from build123d import *

# Parameters (mm, degrees)
F0_W     = 2
F0_H     = 2
F0_W_2   = 1
F0_W_3   = 21
F1_DEPTH = 25
F2_DEPTH = 1
F3_START = 24
F3_DEPTH = 1
F4_W     = 23
F4_H     = 4.75
F5_DEPTH = 25


with BuildPart() as f1:
    # F0 (on Front) → F1 (new body)
    with BuildSketch(Plane.XZ):
        with BuildLine():
            Line((-12.4285714286, 13.5171716937), (-14.4285714286, 13.5171716937))
            Line((-14.4285714286, 13.5171716937), (-14.4285714286, 2.0171716937))
            ThreePointArc((-14.4285714286, 2.0171716937), (-1.9285714286, -10.4828283063), (10.5714285714, 2.0171716937))
            Line((10.5714285714, 2.0171716937), (10.5714285714, 13.5171716937))
            Line((10.5714285714, 13.5171716937), (8.5714285714, 13.5171716937))
            Line((8.5714285714, 13.5171716937), (8.5714285714, 2.0171716937))
            ThreePointArc((8.5714285714, 2.0171716937), (-1.9285714286, -8.4828283063), (-12.4285714286, 2.0171716937))
            Line((-12.4285714286, 2.0171716937), (-12.4285714286, 13.5171716937))
        make_face()
        with Locations((9.5714285714, 14.5171716937)):
            Rectangle(F0_W, F0_H)
        with Locations((-13.4285714286, 14.5171716937)):
            Rectangle(F0_W, F0_H)
        with Locations((-14.9285714286, 14.5171716937)):
            Rectangle(F0_W_2, F0_H)
        with Locations((-1.9285714286, 14.5171716937)):
            Rectangle(F0_W_3, F0_H)
        with Locations((11.0714285714, 14.5171716937)):
            Rectangle(F0_W_2, F0_H)
    extrude(amount=F1_DEPTH)

    # F0 (on Front) → F2 (join)
    with BuildSketch(Plane.XZ):
        with BuildLine():
            Line((-14.4285714286, 13.5171716937), (-15.4285714286, 13.5171716937))
            Line((-15.4285714286, 13.5171716937), (-15.4285714286, 2.0171716937))
            ThreePointArc((-15.4285714286, 2.0171716937), (-11.4745129746, -7.5287698523), (-1.9285714286, -11.4828283063))
            ThreePointArc((-1.9285714286, -11.4828283063), (7.6173701174, -7.5287698523), (11.5714285714, 2.0171716937))
            Line((11.5714285714, 2.0171716937), (11.5714285714, 13.5171716937))
            Line((11.5714285714, 13.5171716937), (10.5714285714, 13.5171716937))
            Line((10.5714285714, 13.5171716937), (10.5714285714, 2.0171716937))
            ThreePointArc((10.5714285714, 2.0171716937), (-1.9285714286, -10.4828283063), (-14.4285714286, 2.0171716937))
            Line((-14.4285714286, 2.0171716937), (-14.4285714286, 13.5171716937))
        make_face()
        with BuildLine():
            Line((-12.4285714286, 13.5171716937), (-14.4285714286, 13.5171716937))
            Line((-14.4285714286, 13.5171716937), (-14.4285714286, 2.0171716937))
            ThreePointArc((-14.4285714286, 2.0171716937), (-1.9285714286, -10.4828283063), (10.5714285714, 2.0171716937))
            Line((10.5714285714, 2.0171716937), (10.5714285714, 13.5171716937))
            Line((10.5714285714, 13.5171716937), (8.5714285714, 13.5171716937))
            Line((8.5714285714, 13.5171716937), (8.5714285714, 2.0171716937))
            ThreePointArc((8.5714285714, 2.0171716937), (-1.9285714286, -8.4828283063), (-12.4285714286, 2.0171716937))
            Line((-12.4285714286, 2.0171716937), (-12.4285714286, 13.5171716937))
        make_face()
        with BuildLine():
            Line((8.5714285714, 13.5171716937), (-12.4285714286, 13.5171716937))
            Line((-12.4285714286, 13.5171716937), (-12.4285714286, 2.0171716937))
            ThreePointArc((-12.4285714286, 2.0171716937), (-1.9285714286, -8.4828283063), (8.5714285714, 2.0171716937))
            Line((8.5714285714, 2.0171716937), (8.5714285714, 13.5171716937))
        make_face()
    extrude(amount=F2_DEPTH)

    # F0 (on Front) → F3 (join)
    with BuildSketch(Plane.XZ.offset(F3_START)):
        with BuildLine():
            Line((-14.4285714286, 13.5171716937), (-15.4285714286, 13.5171716937))
            Line((-15.4285714286, 13.5171716937), (-15.4285714286, 2.0171716937))
            ThreePointArc((-15.4285714286, 2.0171716937), (-11.4745129746, -7.5287698523), (-1.9285714286, -11.4828283063))
            ThreePointArc((-1.9285714286, -11.4828283063), (7.6173701174, -7.5287698523), (11.5714285714, 2.0171716937))
            Line((11.5714285714, 2.0171716937), (11.5714285714, 13.5171716937))
            Line((11.5714285714, 13.5171716937), (10.5714285714, 13.5171716937))
            Line((10.5714285714, 13.5171716937), (10.5714285714, 2.0171716937))
            ThreePointArc((10.5714285714, 2.0171716937), (-1.9285714286, -10.4828283063), (-14.4285714286, 2.0171716937))
            Line((-14.4285714286, 2.0171716937), (-14.4285714286, 13.5171716937))
        make_face()
        with BuildLine():
            Line((-12.4285714286, 13.5171716937), (-14.4285714286, 13.5171716937))
            Line((-14.4285714286, 13.5171716937), (-14.4285714286, 2.0171716937))
            ThreePointArc((-14.4285714286, 2.0171716937), (-1.9285714286, -10.4828283063), (10.5714285714, 2.0171716937))
            Line((10.5714285714, 2.0171716937), (10.5714285714, 13.5171716937))
            Line((10.5714285714, 13.5171716937), (8.5714285714, 13.5171716937))
            Line((8.5714285714, 13.5171716937), (8.5714285714, 2.0171716937))
            ThreePointArc((8.5714285714, 2.0171716937), (-1.9285714286, -8.4828283063), (-12.4285714286, 2.0171716937))
            Line((-12.4285714286, 2.0171716937), (-12.4285714286, 13.5171716937))
        make_face()
        with BuildLine():
            Line((8.5714285714, 13.5171716937), (-12.4285714286, 13.5171716937))
            Line((-12.4285714286, 13.5171716937), (-12.4285714286, 2.0171716937))
            ThreePointArc((-12.4285714286, 2.0171716937), (-1.9285714286, -8.4828283063), (8.5714285714, 2.0171716937))
            Line((8.5714285714, 2.0171716937), (8.5714285714, 13.5171716937))
        make_face()
    extrude(amount=F3_DEPTH)

    # F4 (on face) → F5 (cut, through all)
    with BuildSketch(Plane(origin=(-14.4285714286, 0, 0), x_dir=(0, -1, 0), z_dir=(-1, 0, 0))):
        with Locations((12.5, 11.1421716937)):
            Rectangle(F4_W, F4_H)
    extrude(amount=-F5_DEPTH, mode=Mode.SUBTRACT)


solid = f1.part
Build history of the part. All positions in model axes, mm. A direction names the side the tool comes from. Round coordinates to 2 decimals unless told otherwise and drop trailing zeros. Loops run counter-clockwise (first coordinate to the right, second up) from the corner with the lowest first, then second, coordinate; pieces in that order, holes last. Notation, with made-up numbers: (2.25, -27) -> (32.25, -27) arc R31 ccw to (32.25, 7) -> close; hole circle Ø9 at (75, 12.25). An arc over 180 degrees is marked (long way). One line per item, written item: value. Start each with the question number.
Q1. Cut at B-B on z = 3.5. List the corners of the cut face in (x, y).
Q2. Drop flat-ended pins along their axis: pin 1 Ø3 at (y, z) = (-4, -2) entering from -X; pin 2 Ø7.5 at (y, z) = (-18, 6) entering from +X; pin 3 Ø7.5 at (y, z) = (-8, 6.5) entering from -X. Give the stop position or say it passes through.
Q3. Cut at D-D on x = 8. List the corners of the cut face in (y, z), plus the area to 3 significant figures.
Q4. Cut at C-C on y = -2. List the corners of the cut face in (x, z), plus the area to 3 significant figures.
Q5. Two-plate mould, pull along Y, no slides. Class faces 5 (the face through (-2, 0, 2)), 6 (the face through (-14.429, -12, 5)), 7 (the face through (11.571, -13, 14)): released by +Y, released by -Y, zero draft, split by the parting line, or undercut.
Q6. Probe line 1 along Y through (x, z) = (0, 1.25); line 2 along X through (y, z) = (-11, 4.75); line 3 along Z through (x, y) = (-12.5, -13). List the from-to ranges inside material, lowest first.
Q7. 3-axis set-ups, long thin cutter, end or side, ignore diameter. For faces 1 (the face through (10, -12, 8.767)), 2 (the face through (10.571, -12, 5)), 3 (the face through (8.571, -12, 5)), 4 (the face through (-2.2, -12.34, -10.48)): which of +Z, -Z, +X, -X, +Y, -Y reach the whole face in a straight line?
Q8. Cut at A-A on z = 12.5. List the corners of the cut face in (x, y).
Computed:
1. outline: (-15.43, -25) -> (11.57, -25) -> (11.57, -24) -> (10.57, -24) -> (10.57, -1) -> (11.57, -1) -> (11.57, 0) -> (-15.43, 0) -> (-15.43, -1) -> (-14.43, -1) -> (-14.43, -24) -> (-15.43, -24) -> close; hole (-12.43, -24) -> (8.57, -24) -> (8.57, -1) -> (-12.43, -1) -> close
2. pin 1: x = -14.17
2. pin 2: x = 10.57
2. pin 3: x = -14.43
3. outline: (-25, -7.13) -> (-24, -7.13) -> (-24, -5.58) -> (-1, -5.58) -> (-1, -7.13) -> (0, -7.13) -> (0, 15.52) -> (-25, 15.52) -> close; hole (-24, -1.4) -> (-1, -1.4) -> (-1, 13.52) -> (-24, 13.52) -> close
3. area: 187 mm²
4. outline: (-15.43, 13.52) -> (11.57, 13.52) -> (11.57, 15.52) -> (-15.43, 15.52) -> close; (-14.43, 2.02) arc R12.5 ccw to (10.57, 2.02) -> (10.57, 8.77) -> (8.57, 8.77) -> (8.57, 2.02) arc R10.5 cw to (-12.43, 2.02) -> (-12.43, 8.77) -> (-14.43, 8.77) -> close
4. area: 153 mm²
5. face 5: released by +Y
5. face 6: undercut
5. face 7: zero draft
6. line 1: -25 to -24, -1 to 0
6. line 2: -14.43 to -12.43, 8.57 to 10.57
6. line 3: -4.65 to 8.77, 13.52 to 15.52
7. face 1: +X, -X
7. face 2: -Z, +X
7. face 3: none
7. face 4: -Z
8. outline: (-15.43, -25) -> (11.57, -25) -> (11.57, -24) -> (-15.43, -24) -> close; (-15.43, -1) -> (11.57, -1) -> (11.57, 0) -> (-15.43, 0) -> close
